Autodesk Inventor part; units mm, degrees
ref_plane "YZ Plane" through (0, 0, 0) normal (1, 0, 0) x (0, 1, 0)
ref_plane "XZ Plane" through (0, 0, 0) normal (0, 1, 0) x (-1, 0, 0)
ref_plane "XY Plane" through (0, 0, 0) normal (0, 0, 1) x (1, 0, 0)
sketch "Sketch1" plane through (0, 0, 0) normal (0, 0, 1) x (1, 0, 0)
  line L0 (0, 0) -> (65, 0)
  line L1 (65, 0) -> (65, 45)
  line L2 (65, 45) -> (0, 45)
  line L3 (0, 45) -> (0, 0)
  dimension "d3" = 65
  dimension "d4" = 45
extrude "Extrusion1" add sketch "Sketch1" along normal blind 48
shell "Shell1" thickness 2 removed faces 1 at (43.3333, 45, 16)
sketch "Sketch2" plane through (2, 2, 2) normal (0, 1, 0) x (1, 0, 0)
  line L0 (61, -44) -> (0, -44)
  line L1 (0, -44) -> (10, -44)
  line L2 (10, -44) -> (40, -44)
  line L3 (40, -44) -> (40, -34)
  line L4 (40, -34) -> (10, -34)
  line L5 (10, -34) -> (10, -44)
  line L6 (61, 0) -> (61, -44)
  line L7 (0, -44) -> (0, 0)
  point P0 (-2, 2)
  dimension "d9" = 30
  dimension "d10" = 10
  dimension "d11" = 61
  dimension "d27" = 10
extrude "Extrusion2" cut sketch "Sketch2" against normal through all
sketch "Sketch3" plane through (2, 2, 2) normal (0, 1, 0) x (1, 0, 0)
  line L0 (0, 0) -> (0, -44)
  line L1 (0, -17) -> (0, 33)
  line L2 (0, -17) -> (44, -17)
  line L3 (44, -17) -> (0, -17)
  line L4 (0, -17) -> (0, -19)
  line L5 (0, -19) -> (44, -19)
  line L6 (44, -19) -> (44, -17)
  point P0 (-2, 2)
  dimension "d16" = 44
  dimension "d17" = 2
extrude "Extrusion3" add sketch "Sketch3" along normal blind 26
fillet "Fillet1" radius 4 1 edges at (0, 22.5, 0)
fillet "Fillet2" radius 4 1 edges at (65, 22.5, 0)
fillet "Fillet3" radius 4 1 edges at (65, 22.5, 48)
fillet "Fillet4" radius 4 1 edges at (0, 22.5, 48)
sketch "Sketch4" plane through (2, 2, 2) normal (1, 0, 0) x (0, 0, -1)
  line L0 (-19, 26) -> (-17, 26)
  line L1 (-19, 26) -> (0, 26)
  line L2 (0, 26) -> (0, 28)
  line L3 (0, 28) -> (-19, 28)
  line L4 (-19, 28) -> (-19, 26)
  point P0 (2, -2)
  dimension "d24" = 2
extrude "Extrusion4" add sketch "Sketch4" along normal blind 20
sketch "Sketch8" plane through (2, 2, 2) normal (0, 0, 1) x (1, 0, 0)
  line L0 (0, 43) -> (8, 43)
  line L1 (8, 43) -> (8, 41)
  line L2 (8, 41) -> (0, 41)
  line L3 (0, 41) -> (0, 43)
  point P0 (-2, -2)
  dimension "d28" = 8
  dimension "d29" = 2
extrude "Extrusion5" add sketch "Sketch8" along normal blind 8
sketch "Sketch10" plane through (4, 45, 0) normal (0, 1, 0) x (1, 0, 0)
  line L0 (6, -2) -> (6, -10)
  circle A0 centre (2, -6) radius 1
  point P0 (-4, 0)
extrude "Extrusion7" cut sketch "Sketch10" against normal blind 2
fillet "Fillet6" radius 4 1 edges at (10, 44, 10)
sketch "Sketch13" plane through (63, 45, 46) normal (0, 0, -1) x (-1, 0, 0)
  line L0 (0, -43) -> (0, 0)
  line L1 (0, 0) -> (8, 0)
  line L2 (8, 0) -> (8, -2)
  line L3 (8, -2) -> (0, -2)
  line L4 (0, -2) -> (0, 0)
  point P0 (63, -45)
  point P1 (0, -2)
  dimension "d51" = 8
  dimension "d52" = 2
extrude "Extrusion10" add sketch "Sketch13" along normal blind 8
sketch "Sketch14" plane through (4, 45, 0) normal (0, 1, 0) x (1, 0, 0)
  circle A0 centre (55, -42) radius 1
  point P0 (-4, 0)
extrude "Extrusion11" cut sketch "Sketch14" against normal blind 2
fillet "Fillet7" radius 4 1 edges at (55, 44, 38)
sketch "Sketch15" plane through (4, 0, 0) normal (0, -1, 0) x (1, 0, 0)
  line L0 (57, 0) -> (0, 0)
  line L1 (0, 0) -> (0, 15)
  line L2 (0, 15) -> (57, 15)
  line L3 (57, 15) -> (57, 0)
extrude "Extrusion12" add sketch "Sketch15" along normal blind 15
fillet "Fillet8" radius 10 3 edges at (4, -7.5, 15) (61, -7.5, 15) (32.5, -15, 15)
sketch "Sketch16" plane through (0, 0, 0) normal (0, 0, -1) x (-1, 0, 0)
  line L0 (-41, -15) -> (-24, -15)
  line L1 (-24, -15) -> (-24, -10.2203)
  line L2 (-24, -10.2203) -> (-41, -10.2203)
  line L3 (-41, -10.2203) -> (-41, -15)
  point P0 (0, 0)
  point P1 (-4, -15)
  point P2 (-61, -15)
extrude "Extrusion13" add sketch "Sketch16" along normal blind 15
fillet "Fillet9" radius 7 2 edges at (41, -12.6102, -15) (24, -12.6102, -15)
sketch "Sketch17" plane through (24, -10.2203, 0) normal (0, 1, 0) x (1, 0, 0)
  line L0 (0, 0) -> (8.5, 0)
  circle A0 centre (8.5, 7.5) radius 4
  point P0 (-24, 0)
extrude "Extrusion14" cut sketch "Sketch17" against normal through all
sketch "Sketch19" plane through (2, 2, 46) normal (1, 0, 0) x (0, 0, -1)
  circle A0 centre (22, 35.5) radius 3.125
  point P0 (46, -2)
  point P1 (44, 28)
  dimension "d78" = 6.25
extrude "Extrusion15" cut sketch "Sketch19" against normal through all
properties part number "Bike_Telemetry"
Input: part model. Units: mm. Frame: model coordinates. A direction names the side the tool comes from. Give positions to 0.01 mm unless a question says otherwise; leave off trailing zeros. Loops run counter-clockwise (first coordinate to the right, second up) from the corner with the lowest first, then second, coordinate; pieces in that order, holes last. Notation, with made-up numbers: (13.5, 36) - (31.5, 36) arc R19 cw to (31.5, 69) - close; hole circle Ø6 at (37.5, 71.5). An arc over 180 degrees is marked (long way). Use CSV: the item, a comma, the result in double quotes. Start each with the question number.
Item 1: Section D-D on x = 47. Return loops of the section in (y, z), then the cut area to 3 significant figures.
Item 2: Line query: line 1 (X direction, y = 44.1, z = 6); line 2 (Z direction, x = 9, y = 26.5); line 3 (Z direction, x = 59, y = 44.2). Output: solid intervals per line, ascending.
Item 3: Reachability of faces 1 (the flat face through (61, -7, 3)), 2 (the cylindrical face through (56.141, 43.986, 39.203)), 3 (the flat face through (32, -2, 15)), 4 (the flat face through (5, 43, 5)) from +Z, -Z, +X, -X, +Y, -Y: full face, straight path, thin tool, end or side. Return the list, or none.
Item 4: Section A-A on x = 18. Return loops of the section in (y, z).
Item 5: Mould query, pull axis Z, two halves, no side actions, for faces 5 (the flat face through (10, 44, 4)), 6 (the cylindrical face through (59, -6, 11)), 7 (the cylindrical face through (63.859, 22.815, 1.203)), 8 (the flat face through (0, 23, 24)). Classes: pulls with the +Z half, pulls with the -Z half, needs draft (parallel to the pull), parting line crosses it, or undercut.
Item 6: Section C-C on x = 32.5. Return loops of the section in (y, z), then the cut area to 3 significant figures.
Item 7: Section B-B on y = 24.5. Return loops of the section in (x, z), then the cut area to 3 significant figures.
Item 8: Contact query for flat-ended pins moving along their axis: P1, Ø3, axis at x = 33.5, z = 11.5, coming from the -Y side; P2, Ø5, axis at x = 50.5, z = 17, coming from the +Y side; P3, Ø5, axis at x = 24, z = 8, coming from the +Y side; P4, Ø5, axis at x = 32.5, z = -7.5, coming from the +Y side. Output: stop coordinate, or through.
Ans:
1,outline,"(-15, 0) - (45, 0) - (45, 2) - (2, 2) - (2, 46) - (45, 46) - (45, 48) - (0, 48) - (0, 15) - (-5, 15) arc R10 ccw to (-15, 5) - close"
1,area,"472 mm2"
2,line 1,"x = 0 to 5, 7 to 10, 63 to 65"
2,line 2,"z = 0 to 2, 19 to 21, 46 to 48"
2,line 3,"z = 0 to 2, 38 to 41, 43 to 48"
3,face 1,"+Z, -Z, +X, -Y"
3,face 2,"+Y"
3,face 3,"+Z, +X, -X, -Y"
3,face 4,"none"
4,outline,"(-15, 0) - (45, 0) - (45, 2) - (30, 2) - (30, 21) - (2, 21) - (2, 36) - (0, 36) - (0, 15) - (-5, 15) arc R10 ccw to (-15, 5) - close; (0, 46) - (45, 46) - (45, 48) - (0, 48) - close; hole (2, 2) - (28, 2) - (28, 19) - (2, 19) - close"
5,face 5,"undercut"
5,face 6,"pulls with the +Z half"
5,face 7,"pulls with the -Z half"
5,face 8,"needs draft"
6,outline,"(-15, -15) - (-10.22, -15) - (-10.22, -11.5) - (-15, -11.5) - close; (-15, -3.5) - (-10.22, -3.5) - (-10.22, 0) - (45, 0) - (45, 2) - (2, 2) - (2, 19) - (28, 19) - (28, 21) - (2, 21) - (2, 36) - (0, 36) - (0, 15) - (-5, 15) arc R10 ccw to (-15, 5) - close; (0, 46) - (45, 46) - (45, 48) - (0, 48) - close"
6,area,"537 mm2"
7,outline,"(0, 4) arc R4 ccw to (4, 0) - (61, 0) arc R4 ccw to (65, 4) - (65, 44) arc R4 ccw to (61, 48) - (4, 48) arc R4 ccw to (0, 44) - close; hole (2, 2) - (63, 2) - (63, 46) - (2, 46) - (2, 21) - (46, 21) - (46, 19) - (2, 19) - close"
7,area,"510 mm2"
8,P1,"stops at y = -13.66"
8,P2,"stops at y = 2"
8,P3,"stops at y = 30"
8,P4,"passes through"
